```python
from build123d import *

# Parameters (mm, degrees)
SKETCH1_W           = 1250
SKETCH1_H           = 210.257392811
BOSS_EXTRUDE1_DEPTH = 150
SKETCH2_R           = 75
CUT_EXTRUDE1_DEPTH  = 150
FILLET3_R           = 55
BOSS_EXTRUDE2_DEPTH = 1250


with BuildPart() as part:
    # Sketch1 → Boss-Extrude1 (new body)
    with BuildSketch(Plane.XY):
        with Locations((500, 3.571821645)):
            Rectangle(SKETCH1_W, SKETCH1_H)
    extrude(amount=BOSS_EXTRUDE1_DEPTH)

    # Sketch2 → Cut-Extrude1 (cut)
    with BuildSketch(Plane.XY.offset(150)):
        Circle(SKETCH2_R)
        with Locations((1000, 0)):
            Circle(SKETCH2_R)
    extrude(amount=-CUT_EXTRUDE1_DEPTH, mode=Mode.SUBTRACT)

    # Fillet3
    # the kernel refuses this fillet: 55 mm, written as the material it takes off along each edge
    with BuildSketch(Plane(origin=(1125, 246.20051805, 150), x_dir=(0, 0, -1), z_dir=(0, -1, 0)), Plane(origin=(-125, -239.056874761, 150), x_dir=(0, 0, -1), z_dir=(0, 1, 0))) as fillet3_piece_1:
        with BuildLine():
            CenterArc((FILLET3_R, -FILLET3_R), FILLET3_R, 90, 90)
            Line((0, -FILLET3_R), (0, 0))
            Line((0, 0), (FILLET3_R, 0))
        make_face()
    extrude(amount=485.257392811, mode=Mode.SUBTRACT)
    with BuildSketch(Plane(origin=(1125, 246.20051805, 0), x_dir=(0, 0, 1), z_dir=(0, -1, 0)), Plane(origin=(-125, -239.056874761, 0), x_dir=(0, 0, 1), z_dir=(0, 1, 0))) as fillet3_piece_2:
        with BuildLine():
            CenterArc((FILLET3_R, FILLET3_R), FILLET3_R, 180, 90)
            Line((0, FILLET3_R), (0, 0))
            Line((0, 0), (FILLET3_R, 0))
        make_face()
    extrude(amount=485.257392811, mode=Mode.SUBTRACT)

    # Sketch3 → Boss-Extrude2 (add, through all)
    with BuildSketch(Plane.ZY.offset(125)):
        with BuildLine():
            Line((95, 108.70051805), (55, 108.70051805))
            ThreePointArc((55, 108.70051805), (75, 139.142597248), (95, 108.70051805))
        make_face()
    extrude(amount=-BOSS_EXTRUDE2_DEPTH)


solid = part.part
```
Could you check a few things on this model? Use its own coordinates, in mm. Coordinates: 2 decimals unless noted, no trailing zeros. Write each loop counter-clockwise with the first axis right and the second up, starting at its lowest first coordinate (ties: lowest second). Pieces come first, ordered by that corner, then holes. Notation, with made-up numbers: M 64,1 L 75,1 A26 cw 75,31 Z; hole C -30,42.25 d10. An arc over 180 degrees is marked long. Answer as CSV lines item,"result". Start each with the question number.
1) We'd pull the mould along X, two halves only. Please class faces 1 (the flat face through (492, 5, 0)), 2 (the cylindrical face through (-109.316, 2.1, 133.461)), 3 (the cylindrical face through (-9.764, 74.362, 76.05)): +X half, -X half, draft (parallel to the pull), parting line (faces both ways), or undercut.
2) Please list where these lines run through material, in increasing order: line 1 (X direction, y = 0, z = 83); line 2 (X direction, y = -65, z = 90.5); line 3 (Y direction, x = 1000, z = 47). Write a range as from..to.
3) I want a section at D-D, the plane x = 556. Please give me the cut outline in (y, z).
4) For P1, Ø2, axis at x = 600, z = 52, coming from the +Y side; P2, Ø3, axis at x = 691, y = 74.5, coming from the -Z side; P3, Ø4, axis at y = -27.5, z = 115.5, coming from the -X side; P4, Ø8, axis at y = 50.5, z = 15.5, coming from the +X side, each with a flat end and sliding along its axis, tell me the tip position at first contact or that it passes through.
5) I want a section at C-C, the plane y = -41.5. Please give me the cut outline in (x, z).
6) I want a section at A-A, the plane x = 0. Please give me the cut outline in (y, z).
7) I want a section at B-B, the plane z = 75. Please give me the cut outline in (x, y), and give its area (3 significant figures).
Data:
1,face 1,"draft"
1,face 2,"-X half"
1,face 3,"undercut"
2,line 1,"x = -125..-75, 75..925, 1075..1125"
2,line 2,"x = -125..-37.42, 37.42..962.58, 1037.42..1125"
2,line 3,"y = -101.56..-75, 75..108.7"
3,outline,"M -101.56,0 L 108.7,0 L 108.7,55 A21.79 ccw long 108.7,95 L 108.7,150 L -101.56,150 Z"
4,P1,"stops at y = 108.7"
4,P2,"stops at z = 0"
4,P3,"stops at x = -121.8"
4,P4,"stops at x = 1112.01"
5,outline,"M -125,55 A55 ccw -70,0 L -62.47,0 L -62.47,150 L -70,150 A55 ccw -125,95 Z; M 62.47,0 L 937.53,0 L 937.53,150 L 62.47,150 Z; M 1062.47,0 L 1070,0 A55 ccw 1125,55 L 1125,95 A55 ccw 1070,150 L 1062.47,150 Z"
6,outline,"M -101.56,0 L -75,0 L -75,150 L -101.56,150 Z; M 75,0 L 108.7,0 L 108.7,55 A21.79 ccw long 108.7,95 L 108.7,150 L 75,150 Z"
7,outline,"M -125,-101.56 L 1125,-101.56 L 1125,139.14 L -125,139.14 Z; hole C 0,0 d150; hole C 1000,0 d150"
7,area,"266,000 mm^2"
